Autodesk Inventor part; units mm, degrees
ref_plane "Work Plane1" through (0, 125, 0) normal (0, 1, 0) x (-1, 0, 0)
ref_plane "YZ Plane" through (0, 0, 0) normal (1, 0, 0) x (0, 1, 0)
ref_plane "XY Plane" through (0, 0, 0) normal (0, 0, 1) x (1, 0, 0)
sketch "Sketch1" plane through (0, 0, 0) normal (0, 0, 1) x (1, 0, 0)
  line L0 (-62, 0) -> (-62, 87)
  arc A0 (-27, 122) -> (-62, 87) centre (-27, 87) ccw
  line L1 (-27, 122) -> (27, 122)
  arc A1 (62, 87) -> (27, 122) centre (27, 87) ccw
  line L2 (62, 87) -> (62, 0)
  point P0 (0, 0)
  point P1 (0, 122)
  point P2 (62, 43.5)
  dimension "d0" = 122
  dimension "d1" = 124
  dimension "d2" = 35
sketch "Sketch2" plane through (0, 0, 0) normal (0, 1, 0) x (-1, 0, 0)
  line L0 (62, 4) -> (62, -4)
  line L1 (62, -4) -> (40, -4)
  line L2 (40, -4) -> (40, -14)
  line L3 (40, -14) -> (32, -14)
  line L4 (32, -14) -> (32, 14)
  line L5 (32, 14) -> (40, 14)
  line L6 (40, 14) -> (40, 4)
  line L7 (40, 4) -> (62, 4)
  point P0 (0, 0)
  point P1 (62, 0)
  point P2 (32, 0)
  point P3 (62, 0)
  dimension "d4" = 30
  dimension "d5" = 28
  dimension "d6" = 8
  dimension "d7" = 8
sweep "Sweep1" add profiles "Sketch2" path "Sketch1"
sketch "Sketch3" plane through (0, 0, 0) normal (0, 1, 0) x (-1, 0, 0)
  line L0 (-40, -28) -> (-62, -28)
  line L1 (-62, -28) -> (-62, 28)
  line L2 (-62, 28) -> (-40, 28)
  line L3 (-40, 28) -> (-40, -28)
  line L4 (-62, -4) -> (-62, 4)
  point P0 (0, 0)
  point P1 (-62, 0)
  dimension "d10" = 22
  dimension "d11" = 56
extrude "Extrusion1" add sketch "Sketch3" along normal blind 17
fillet "Fillet1" radius 3 4 edges at (62, 8.5, 28) (40, 8.5, 28) (62, 8.5, -28) (40, 8.5, -28)
sketch "Sketch4" plane through (0, 17, 0) normal (0, 1, 0) x (1, 0, 0)
  line L0 (43, -28) -> (59, -28)
  line L1 (51, 17) -> (51, -17) construction
  point P0 (0, 0)
  point P1 (51, 0)
  point P2 (51, -28)
  dimension "d15" = 34
hole "Hole1" at (51, 17, -17) at (51, 17, 17) direction (0, -1, 0) diameter 11 end through all
mirror "Mirror1" about plane through (0, 0, 0) normal (1, 0, 0) of "Extrusion1", "Fillet1", "Hole1"
ref_plane "Work Plane1" through (0, 125, 0) normal (0, 1, 0) x (-1, 0, 0)
sketch "Sketch5" plane through (0, 125, 0) normal (0, 1, 0) x (-1, 0, 0)
  circle A0 centre (0, 0) radius 18.5
  dimension "d24" = 37
extrude "Extrusion2" add sketch "Sketch5" against normal blind 40
sketch "Sketch6" plane through (0, 125, 0) normal (0, 1, 0) x (1, 0, 0)
  circle A0 centre (0, 0) radius 18.5
hole "Hole2" at (0, 125, 0) direction (0, -1, 0) diameter 20 end through all
properties part number "Part029. Shaft guide" material "Steel, Cast"
Can you work these out from the model? Positions are in its coordinate system, mm. A direction names the side the tool comes from. Round coordinates to 2 decimals unless told otherwise and drop trailing zeros. Write each loop counter-clockwise with the first axis right and the second up, starting at its lowest first coordinate (ties: lowest second). Pieces come first, ordered by that corner, then holes. Notation, with made-up numbers: (56.5, 9.25) - (100.5, 9.25) arc R19 ccw to (100.5, 44.25) - close; hole circle Ø2 at (13, 55). An arc over 180 degrees is marked (long way). Write each question's results on one line, items separated by ' | '. Start each with the question number.
1) Suppose I cut it at B-B (x = 54). List the corners of the cut face in (y, z) for me, and give its area (3 significant figures).
2) Which directions (+Z, -Z, +X, -X, +Y, -Y) give clear straight access to the entire face, cutting with the end or side of a thin tool? Please do faces 5 (the cylindrical face through (-40.86, 8.62, -27.1)), 6 (the cylindrical face through (-17.089, 105.28, -7.086)), 7 (the cylindrical face through (-36.091, 96.293, 9.07)), 8 (the cylindrical face through (30, 91, 0)), 9 (the flat face through (-45, 82, -4)).
3) We'd pull the mould along X, two halves only. Please class faces 1 (the flat face through (-40, 8, -20)), 2 (the flat face through (-51, 8, 28)), 3 (the flat face through (40, 52, 9)), 4 (the cylindrical face through (-56.453, 8.381, 16.284)): released by +X, released by -X, zero draft, split by the parting line, or undercut.
4) Suppose I cut it at C-C (x = 1.5). List the corners of the cut face in (y, z) for me.
5) Please list where these lines run through material, in increasing order: line 1 (X direction, y = 8, z = 17); line 2 (Z direction, x = 51, y = 11); line 3 (Z direction, x = 0, y = 98).
6) Suppose I cut it at A-A (z = 0). List the corners of the cut face in (x, y) for me, and give its area (3 significant figures).
7) Suppose I cut it at D-D (z = 17). List the corners of the cut face in (x, y) for me.
8) For pin 1 Ø12 at (y, z) = (100, 10.5) entering from -X; pin 2 Ø16.5 at (x, z) = (23, 4) entering from -Y; pin 3 Ø4 at (x, z) = (24.5, 1.5) entering from +Y, each with a flat end and sliding along its axis, tell me the tip position at first contact or that it passes through.
Here are the results:
1) outline: (0, -28) - (17, -28) - (17, -21.61) - (0, -21.61) - close; (0, -12.39) - (17, -12.39) - (17, -4) - (109.27, -4) - (109.27, 4) - (17, 4) - (17, 12.39) - (0, 12.39) - close; (0, 21.61) - (17, 21.61) - (17, 28) - (0, 28) - close | area: 1,380 mm2
2) face 5: -Z, +Y, -Y | face 6: none | face 7: +Z, -X, +Y | face 8: +Z, -Z, -Y | face 9: -Z, -X, +Y
3) face 1: undercut | face 2: zero draft | face 3: released by +X | face 4: undercut
4) outline: (85, -18.44) - (125, -18.44) - (125, -9.89) - (85, -9.89) - close; (85, 9.89) - (125, 9.89) - (125, 18.44) - (85, 18.44) - close
5) line 1: x = -62 to -56.5, -45.5 to -40, 40 to 45.5, 56.5 to 62 | line 2: z = -28 to -22.5, -11.5 to 11.5, 22.5 to 28 | line 3: z = -18.5 to -10, 10 to 18.5
6) outline: (-62, 0) - (-32, 0) - (-32, 87) arc R5 cw to (-27, 92) - (-18.5, 92) - (-18.5, 85) - (-10, 85) - (-10, 125) - (-18.5, 125) - (-18.5, 122) - (-27, 122) arc R35 ccw to (-62, 87) - close; (10, 85) - (18.5, 85) - (18.5, 92) - (27, 92) arc R5 cw to (32, 87) - (32, 0) - (62, 0) - (62, 87) arc R35 ccw to (27, 122) - (18.5, 122) - (18.5, 125) - (10, 125) - close | area: 8,290 mm2
7) outline: (-62, 0) - (-56.5, 0) - (-56.5, 17) - (-62, 17) - close; (-45.5, 0) - (-40, 0) - (-40, 17) - (-45.5, 17) - close; (-7.3, 85) - (7.3, 85) - (7.3, 125) - (-7.3, 125) - close; (40, 0) - (45.5, 0) - (45.5, 17) - (40, 17) - close; (56.5, 0) - (62, 0) - (62, 17) - (56.5, 17) - close
8) pin 1: stops at x = -37.95 | pin 2: stops at y = 85 | pin 3: stops at y = 122
